```python
from build123d import *

# Parameters (mm, degrees)
SKETCH1_R           = 50.8
BOSS_EXTRUDE2_DEPTH = 30
SKETCH3_R           = 44.45
CUT_EXTRUDE1_DEPTH  = 25
SKETCH4_R           = 2.794
BOSS_EXTRUDE3_DEPTH = 25
SKETCH5_R           = 2.54
CUT_EXTRUDE2_DEPTH  = 25


with BuildPart() as part:
    # Sketch1 → Boss-Extrude2 (new body)
    with BuildSketch(Plane(origin=(0, 0, 0), x_dir=(1, 0, 0), z_dir=(0, 1, 0))):
        Circle(SKETCH1_R)
    extrude(amount=BOSS_EXTRUDE2_DEPTH)

    # Sketch3 → Cut-Extrude1 (cut)
    with BuildSketch(Plane(origin=(0, 30, 0), x_dir=(1, 0, 0), z_dir=(0, 1, 0))):
        Circle(SKETCH3_R)
    extrude(amount=-CUT_EXTRUDE1_DEPTH, mode=Mode.SUBTRACT)

    # Sketch4 → Boss-Extrude3 (add)
    with BuildSketch(Plane(origin=(0, 5, 0), x_dir=(1, 0, 0), z_dir=(0, 1, 0))):
        Circle(SKETCH4_R)
    extrude(amount=BOSS_EXTRUDE3_DEPTH)

    # Sketch5 → Cut-Extrude2 (cut)
    with BuildSketch(Plane(origin=(0, 30, 0), x_dir=(1, 0, 0), z_dir=(0, 1, 0))):
        Circle(SKETCH5_R)
    extrude(amount=-CUT_EXTRUDE2_DEPTH, mode=Mode.SUBTRACT)


solid = part.part
```
CAD build for the part. Positions are in the model's coordinates, mm. A direction names the side the tool comes from. Coordinates: 2 decimals unless noted, no trailing zeros. Write each loop counter-clockwise with the first axis right and the second up, starting at its lowest first coordinate (ties: lowest second). Pieces come first, ordered by that corner, then holes. Notation, with made-up numbers: (60, 53) -> (119, 53) arc R22 cw to (119, 86) -> close; hole circle Ø4 at (-16, 29). An arc over 180 degrees is marked (long way). Return JSON: item names as keys, results as strings. Group by question number.
Q1. Drill centre lines: line 1 (X direction, y = 11.5, z = 0); line 2 (Z direction, x = 1, y = 14.25). Where is each one in solid material? Low to high.
Q2. Flat gauge pins, fed straight in: pin 1 (6 mm diameter, centred on y = 6, z = -1.5, fed in from -X); pin 2 (4 mm diameter, centred on y = 25.5, z = 33, fed in from +X); pin 3 (12 mm diameter, centred on x = -4.5, y = 18, fed in from -Z); pin 4 (10 mm diameter, centred on x = -4, y = 26.5, fed in from +Z). Where does each tip first touch, or does it go through?
Q3. Cut at A-A, the plane y = 15.5. Give the cut face in (x, z), then the cut area to 3 significant figures.
Q4. Cut at D-D, the plane z = 39. Give the cut face in (x, y).
Q5. Cut at B-B, the plane z = 0. Give the cut face in (x, y), then the cut area to 3 significant figures.
Q6. Cut at C-C, the plane x = 0. Give the cut face in (y, z).
Q7. Which spindle directions (+Z, -Z, +X, -X, +Y, -Y) get a long thin tool onto all of the face, cutting with end or side? Do faces 4 (the face through (-2.217, 17.325, 1.7)), 5 (the face through (-1, 0, -1)). Say none if no direction does.
Q8. Pull direction Z, two halves, no side cores. Call faces 1 (the face through (-11.012, 14.79, 49.592)), 2 (the face through (42.397, 17.675, -13.352)), 3 (the face through (0, 30, 45)): released by +Z, released by -Z, zero draft, split by the parting line, or undercut.
Returned:
{
 "1": {"line 1": "x = -50.8 to -44.45, -2.79 to -2.54, 2.54 to 2.79, 44.45 to 50.8", "line 2": "z = -50.79 to -44.44, -2.61 to -2.33, 2.33 to 2.61, 44.44 to 50.79"},
 "2": {"pin 1": "stops at x = -50.8", "pin 2": "stops at x = 40.24", "pin 3": "stops at z = -50.8", "pin 4": "stops at z = 50.8"},
 "3": {"outline": "circle Ø101.6 at (0, 0); circle Ø5.59 at (0, 0); hole circle Ø88.9 at (0, 0); hole circle Ø5.08 at (0, 0)", "area": "1,900 mm2"},
 "4": {"outline": "(-32.55, 0) -> (32.55, 0) -> (32.55, 30) -> (21.33, 30) -> (21.33, 5) -> (-21.33, 5) -> (-21.33, 30) -> (-32.55, 30) -> close"},
 "5": {"outline": "(-50.8, 0) -> (50.8, 0) -> (50.8, 30) -> (44.45, 30) -> (44.45, 5) -> (2.79, 5) -> (2.79, 30) -> (2.54, 30) -> (2.54, 5) -> (-2.54, 5) -> (-2.54, 30) -> (-2.79, 30) -> (-2.79, 5) -> (-44.45, 5) -> (-44.45, 30) -> (-50.8, 30) -> close", "area": "838 mm2"},
 "6": {"outline": "(0, -50.8) -> (30, -50.8) -> (30, -44.45) -> (5, -44.45) -> (5, -2.79) -> (30, -2.79) -> (30, -2.54) -> (5, -2.54) -> (5, 2.54) -> (30, 2.54) -> (30, 2.79) -> (5, 2.79) -> (5, 44.45) -> (30, 44.45) -> (30, 50.8) -> (0, 50.8) -> close"},
 "7": {"face 4": "+Y", "face 5": "+Z, -Z, +X, -X, -Y"},
 "8": {"face 1": "split by the parting line", "face 2": "undercut", "face 3": "zero draft"}
}
